from build123d import *

# Parameters (mm, degrees)
DODANIE_WYCI_GNI_CIE1_DEPTH = 850
SZKIC3_W                    = 183.44852115
SZKIC3_H                    = 118.68309716
WYTNIJ_WYCI_GNI_CIE1_DEPTH  = 605.02814504


with BuildPart() as part:
    # Szkic2 → Dodanie-wyciągnięcie1 (new body)
    with BuildSketch(Plane.XY):
        with BuildLine():
            ThreePointArc((0, 57), (0.878679656, 59.121320344), (3, 60))
            Line((3, 60), (57, 60))
            ThreePointArc((57, 60), (59.121320344, 59.121320344), (60, 57))
            Line((60, 57), (60, 3))
            ThreePointArc((60, 3), (59.121320344, 0.878679656), (57, 0))
            Line((57, 0), (3, 0))
            ThreePointArc((3, 0), (0.878679656, 0.878679656), (0, 3))
            Line((0, 3), (0, 57))
        make_face()
        with BuildLine():
            Line((3, 6), (3, 54))
            ThreePointArc((3, 54), (3.878679656, 56.121320344), (6, 57))
            Line((6, 57), (54, 57))
            ThreePointArc((54, 57), (56.121320344, 56.121320344), (57, 54))
            Line((57, 54), (57, 6))
            ThreePointArc((57, 6), (56.121320344, 3.878679656), (54, 3))
            Line((54, 3), (6, 3))
            ThreePointArc((6, 3), (3.878679656, 3.878679656), (3, 6))
        make_face(mode=Mode.SUBTRACT)
    extrude(amount=DODANIE_WYCI_GNI_CIE1_DEPTH)

    # Szkic3 → Wytnij-wyciągnięcie1 (cut, through all)
    with BuildSketch(Plane(origin=(425, 0, 425), x_dir=(0, 1, 0), z_dir=(0.7071067811865488, 0, 0.7071067811865464))):
        with Locations((36.943590896, 573.417053453)):
            Rectangle(SZKIC3_W, SZKIC3_H)
    extrude(amount=WYTNIJ_WYCI_GNI_CIE1_DEPTH, mode=Mode.SUBTRACT)


solid = part.part
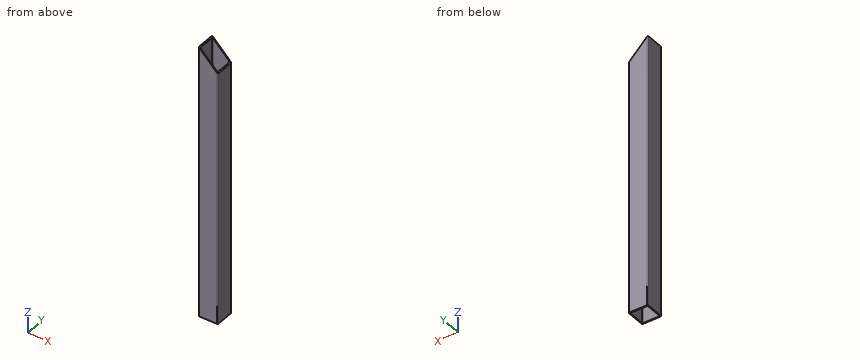
Work out the finished part from the listing and answer in its coordinate system (mm). Give positions to 0.01 mm unless a question says otherwise; leave off trailing zeros. Loops run counter-clockwise (first coordinate to the right, second up) from the corner with the lowest first, then second, coordinate; pieces in that order, holes last. Notation, with made-up numbers: (-15, 83.5) -> (43, 83.5) arc R11 cw to (43, 88.5) -> close; hole circle Ø9 at (-20, 7). An arc over 180 degrees is marked (long way). Use a Markdown table: item, result. Add a question column.
1. Section C-C on z = 287.5 is taken. Determine the outline of the cut face in (x, y), and give its area (3 significant figures).
2. Section B-B on y = 29.5 is taken. Determine the outline of the cut face in (x, z), and give its area (3 significant figures).
3. Section A-A on x = 39 is taken. Determine the outline of the cut face in (y, z).
4. Find the intervals of material crossed by probe 1 along Y at (x, z) = (18.5, 534); probe 2 along Y at (x, z) = (55.5, 562), in increasing order.
Results below:
| question | item | result |
|---|---|---|
| 1 | outline | (0, 3) arc R3 ccw to (3, 0) -> (57, 0) arc R3 ccw to (60, 3) -> (60, 57) arc R3 ccw to (57, 60) -> (3, 60) arc R3 ccw to (0, 57) -> close; hole (3, 6) arc R3 ccw to (6, 3) -> (54, 3) arc R3 ccw to (57, 6) -> (57, 54) arc R3 ccw to (54, 57) -> (6, 57) arc R3 ccw to (3, 54) -> close |
| 1 | area | 684 mm^2 |
| 2 | outline | (0, 0) -> (3, 0) -> (3, 847) -> (0, 850) -> close; (57, 0) -> (60, 0) -> (60, 790) -> (57, 793) -> close |
| 2 | area | 4,920 mm^2 |
| 3 | outline | (0, 0) -> (3, 0) -> (3, 811) -> (0, 811) -> close; (57, 0) -> (60, 0) -> (60, 811) -> (57, 811) -> close |
| 4 | probe 1 | y = 0 to 3, 57 to 60 |
| 4 | probe 2 | y = 0 to 3.4, 56.6 to 60 |
